from build123d import *

# Parameters (mm, degrees)
SKETCH1_R               = 3.048
SKETCH1_W               = 3.175
SKETCH1_H               = 8.7376
BOSS_EXTRUDE1_DEPTH     = 17.78
SKETCH3_W               = 3.937
SKETCH3_H               = 8.7376
BOSS_EXTRUDE2_DEPTH     = 3.175
SKETCH5_R               = 1.651
SKETCH5_R_2             = 3.048
BOSS_EXTRUDE3_DEPTH     = 17.78
FILLET1_R               = 31.75
FILLET2_R               = 1.27
SKETCH2_R               = 2.159
CUT_EXTRUDE2_DEPTH      = 12.7
CUT_EXTRUDE3_DEPTH      = 45.217979663
CUT_EXTRUDE3_DEPTH_BACK = 45.217979663
SKETCH7_W               = 24.098797772
SKETCH7_H               = 63.864925988
SKETCH7_W_2             = 12.7
SKETCH7_H_2             = 50.8


with BuildPart() as part:
    # Sketch1 → Boss-Extrude1 (new body)
    with BuildSketch(Plane.XY):
        with BuildLine():
            Line((-12.065, 8.128), (-1.27, 8.128))
            Line((-1.27, 8.128), (3.448633975, 4.557208434))
            ThreePointArc((3.448633975, 4.557208434), (5.712149959, 0.180465622), (3.72942373, -4.33042996))
            Line((3.72942373, -4.33042996), (-1.27, -8.2296))
            Line((-1.27, -8.2296), (-12.065, -8.2296))
            Line((-12.065, -8.2296), (-12.065, 8.128))
        make_face()
        Circle(SKETCH1_R, mode=Mode.SUBTRACT)
        with Locations((-6.6675, -0.0508)):
            Rectangle(SKETCH1_W, SKETCH1_H, mode=Mode.SUBTRACT)
    extrude(amount=BOSS_EXTRUDE1_DEPTH)

    # Sketch3 → Boss-Extrude2 (add)
    with BuildSketch(Plane.ZY.offset(5.08)):
        with Locations((1.9685, -0.0508)):
            Rectangle(SKETCH3_W, SKETCH3_H)
    extrude(amount=BOSS_EXTRUDE2_DEPTH)

    # Sketch5 → Boss-Extrude3 (add)
    with BuildSketch(Plane(origin=(0, 0, 0), x_dir=(-1, 0, 0), z_dir=(0, 0, -1))):
        with BuildLine():
            Line((-2.932939367, 5.08), (4.490590949, 17.937931679))
            ThreePointArc((4.490590949, 17.937931679), (11.43, 19.797340731), (13.289409051, 12.857931679))
            Line((13.289409051, 12.857931679), (8.652171134, 4.826))
            Line((8.652171134, 4.826), (5.08, 4.826))
            Line((5.08, 4.826), (5.08, -4.4196))
            Line((5.08, -4.4196), (8.417535985, -4.4196))
            Line((8.417535985, -4.4196), (13.289409051, -12.857931679))
            ThreePointArc((13.289409051, -12.857931679), (11.43, -19.797340731), (4.490590949, -17.937931679))
            Line((4.490590949, -17.937931679), (-2.932939367, -5.08))
            Line((-2.932939367, -5.08), (-17.78, -5.08))
            ThreePointArc((-17.78, -5.08), (-22.86, 0), (-17.78, 5.08))
            Line((-17.78, 5.08), (-2.932939367, 5.08))
        make_face()
        with Locations((8.89, 15.397931679)):
            Circle(SKETCH5_R, mode=Mode.SUBTRACT)
        with Locations((8.89, -15.397931679)):
            Circle(SKETCH5_R, mode=Mode.SUBTRACT)
        with Locations((-17.78, 0)):
            Circle(SKETCH5_R, mode=Mode.SUBTRACT)
        with Locations(Location((0, 0, 0), (0, 0, 180))):
            Circle(SKETCH5_R_2, mode=Mode.SUBTRACT)
    extrude(amount=-BOSS_EXTRUDE3_DEPTH)

    # Fillet1
    fillet1_edges = [part.edges().sort_by_distance(p)[0] for p in [
        (2.932939367, -5.08, 8.89),
        (2.932939367, 5.08, 8.89),
    ]]
    fillet(fillet1_edges, radius=FILLET1_R)

    # Fillet2
    # the kernel refuses this fillet: 1.27 mm, written as the material it adds along each edge
    with BuildSketch(Plane(origin=(-10.558581723, 8.128, 17.78), x_dir=(-0.4999999999999911, 0.8660254037844438, 0), z_dir=(0, 0, -1))) as fillet2_piece_1:
        with BuildLine():
            CenterArc((2.022737824, -1.27), FILLET2_R, 90, 91.561006687)
            Line((0.753209139, -1.304596497), (0.727818565, -1.305288427))
            ThreePointArc((0.727818565, -1.305288427), (0.354607524, -0.664998248), (-0.021997045, -0.0127))
            Line((-0.021997045, -0.0127), (0, 0.0254))
            Line((0, 0.0254), (2.022737824, 0.0254))
            Line((2.022737824, 0.0254), (2.022737824, 0))
        make_face()
    extrude(amount=17.78)
    with BuildSketch(Plane(origin=(-10.61724051, -8.2296, 0), x_dir=(-1, 0, 0), z_dir=(0, 0, 1))) as fillet2_piece_2:
        with BuildLine():
            CenterArc((2.096740449, 1.091660989), FILLET2_R, 150, 89.268962563)
            Line((0.996888187, 1.726660989), (0.974891141, 1.739360989))
            Line((0.974891141, 1.739360989), (-0.021997045, 0.0127))
            Line((-0.021997045, 0.0127), (0, -0.0254))
            ThreePointArc((0, -0.0254), (0.723879745, -0.0254), (1.434779871, -0.02183322))
            Line((1.434779871, -0.02183322), (1.44775949, 0))
        make_face()
    extrude(amount=17.78)

    # Sketch2 → Cut-Extrude2 (cut)
    with BuildSketch(Plane.ZY.offset(12.065)):
        with Locations(Location((8.89, -0.0508, 0), (0, 0, 270))):
            Circle(SKETCH2_R)
    extrude(amount=-CUT_EXTRUDE2_DEPTH, mode=Mode.SUBTRACT)

    # Sketch7 → Cut-Extrude3 (cut, two sides: drawn at the far end of the back side and taken through both)
    with BuildSketch(Plane.ZY.offset(12.065).offset(-CUT_EXTRUDE3_DEPTH_BACK)):
        with Locations((8.89, -0.0508)):
            Rectangle(SKETCH7_W, SKETCH7_H)
        with Locations((8.89, -0.0508)):
            Rectangle(SKETCH7_W_2, SKETCH7_H_2, mode=Mode.SUBTRACT)
    extrude(amount=CUT_EXTRUDE3_DEPTH + CUT_EXTRUDE3_DEPTH_BACK, mode=Mode.SUBTRACT)


solid = part.part
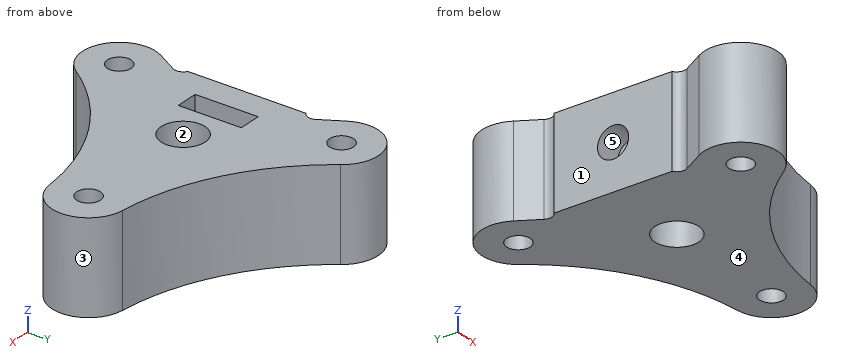
Geometry: final body of the model. Coordinates: model frame, mm. Face numbers are marked on the shaded views. A direction names the side the tool comes from. Give positions to 0.01 mm unless a question says otherwise; leave off trailing zeros. Write each loop counter-clockwise with the first axis right and the second up, starting at its lowest first coordinate (ties: lowest second). Pieces come first, ordered by that corner, then holes. Notation, with made-up numbers: (-23, 53) -> (22, 53) arc R31 cw to (22, 87) -> close; hole circle Ø5 at (63.25, 46). An arc over 180 degrees is marked (long way). Answer in a Markdown table with one row per item.
(1) Ray query, line 1 along X through (y, z) = (-2.5, 6) (3 decimals); line 2 along Y through (x, z) = (-7.5, 8.75); line 3 along Y through (x, z) = (-8.89, 8.5). Return the intervals inside material, ascending. Write a range as [from, to].
Answers below:
| item | result |
|---|---|
| line 1 | [-12.065, -8.255], [-5.08, -1.744], [1.744, 22.202] |
| line 2 | [-20.28, -16.29], [-14.51, -4.42], [4.32, 14.51], [16.29, 20.28] |
| line 3 | [-20.48, -17.05], [-13.75, -2.17], [2.07, 13.75], [17.05, 20.48] |
(2) Section query B-B on y = 0. Return loops of the section in (x, z) (3 decimals), then the cut area to 3 significant figures.
Answers below:
| item | result |
|---|---|
| outline | (-12.065, 2.54) -> (-3.048, 2.54) -> (-3.048, 6.732) -> (-5.08, 6.732) -> (-5.08, 3.937) -> (-8.255, 3.937) -> (-8.255, 6.732) -> (-12.065, 6.732) -> close; (-12.065, 11.048) -> (-8.255, 11.048) -> (-8.255, 15.24) -> (-12.065, 15.24) -> close; (-5.08, 11.048) -> (-3.048, 11.048) -> (-3.048, 15.24) -> (-5.08, 15.24) -> close; (3.048, 2.54) -> (16.129, 2.54) -> (16.129, 15.24) -> (3.048, 15.24) -> close; (19.431, 2.54) -> (22.86, 2.54) -> (22.86, 15.24) -> (19.431, 15.24) -> close |
| area | 263 mm^2 |
(3) Pin query (flat end, axial travel): pin 1 (1.5 mm diameter, centred on x = 11.5, z = 10, fed in from -Y); pin 2 (1 mm diameter, centred on x = -7, y = 0, fed in from +Z); pin 3 (10 mm diameter, centred on x = 16.5, y = -11, fed in from -Z); pin 4 (5 mm diameter, centred on y = -0.05, z = 8.89, fed in from -X) (3 decimals). Return the tip coordinate at first contact, or that it passes through.
Answers below:
| item | result |
|---|---|
| pin 1 | y = -6.68 |
| pin 2 | z = 3.94 |
| pin 3 | through |
| pin 4 | x = -12.065 |
(4) Section query C-C on z = 4.5. State how many separate pieces and enclosed holes the cut face has, then the cut area to 3 significant figures.
Answers below:
| item | result |
|---|---|
| separate pieces | 1 |
| enclosed holes | 5 |
| area | 699 mm^2 |
(5) Set-up query: the marked faces 1 and 2. Return all of +Z, -Z, +X, -X, +Y, -Y with unobstructed straight access to the full face (end or side cutting, diameter ignored); none if empty.
Answers below:
| item | result |
|---|---|
| face 1 | +Z, -Z, -X |
| face 2 | +Z, -Z |
(6) Draft query along Y for the marked faces 3, 4 and 5. Return one class per face: +Y half, -Y half, draft (parallel to the pull), parting line (faces both ways), or undercut.
Answers below:
| item | result |
|---|---|
| face 3 | parting line |
| face 4 | draft |
| face 5 | undercut |
(7) Section query A-A on x = -8.89. Return loops of the section in (y, z).
Answers below:
| item | result |
|---|---|
| outline | (-20.48, 2.54) -> (-17.05, 2.54) -> (-17.05, 15.24) -> (-20.48, 15.24) -> close; (-13.75, 2.54) -> (13.75, 2.54) -> (13.75, 15.24) -> (-13.75, 15.24) -> close; (17.05, 2.54) -> (20.48, 2.54) -> (20.48, 15.24) -> (17.05, 15.24) -> close; hole circle Ø4.32 at (-0.05, 8.89) |
